Part model, mm, in its own coordinate system. A direction names the side the tool comes from. Coordinates: 2 decimals unless noted, no trailing zeros. Order: outer loops, then holes, each group sorted by start corner. A loop starts at its lowest first (then second) coordinate and runs counter-clockwise, first axis right, second up.
from build123d import *

# Parameters (mm, degrees)
F0_R           = 4.75
F1_DEPTH       = 2.5
F2_D           = 4.25
F3_D           = 4.5
F3_CSINK_D     = 7
F3_CSINK_ANGLE = 90
F4_D           = 4
F4_CBORE_D     = 7
F4_CBORE_DEPTH = 1


with BuildPart() as f1:
    # F0 (on Front) → F1 (new body)
    with BuildSketch(Plane.XZ):
        with BuildLine():
            ThreePointArc((60.5, 28.5), (59.62132, 30.62132), (57.5, 31.5))
            Line((57.5, 31.5), (-57.5, 31.5))
            ThreePointArc((-57.5, 31.5), (-59.62132, 30.62132), (-60.5, 28.5))
            Line((-60.5, 28.5), (-60.5, -28.5))
            ThreePointArc((-60.5, -28.5), (-59.62132, -30.62132), (-57.5, -31.5))
            Line((-57.5, -31.5), (57.5, -31.5))
            ThreePointArc((57.5, -31.5), (59.62132, -30.62132), (60.5, -28.5))
            Line((60.5, -28.5), (60.5, 28.5))
        make_face()
        with Locations((-44.260606, 0)):
            Circle(F0_R, mode=Mode.SUBTRACT)
        with BuildLine():
            ThreePointArc((11.989579, 27.5), (25.096687, 16.436433), (30, 0))
            ThreePointArc((30, 0), (25.096687, -16.436433), (11.989579, -27.5))
            ThreePointArc((11.989579, -27.5), (0, -30), (-11.989579, -27.5))
            ThreePointArc((-11.989579, -27.5), (-30, 0), (-11.989579, 27.5))
            ThreePointArc((-11.989579, 27.5), (0, 30), (11.989579, 27.5))
        make_face(mode=Mode.SUBTRACT)
        with BuildLine():
            Line((-11.989579, 27.5), (11.989579, 27.5))
            ThreePointArc((11.989579, 27.5), (0, 30), (-11.989579, 27.5))
        make_face()
        with BuildLine():
            ThreePointArc((-11.989579, -27.5), (0, -30), (11.989579, -27.5))
            Line((11.989579, -27.5), (-11.989579, -27.5))
        make_face()
    extrude(amount=F1_DEPTH)

    # F2 (through all)
    with Locations(Plane(origin=(0, 0, 0), x_dir=(1, 0, 0), z_dir=(0, 1, 0))):
        with Locations((-56.5, 25.75), (56.5, 25.75), (56.5, -25.75), (-56.5, -25.75)):
            Hole(F2_D / 2)

    # F3 (through all)
    with Locations(Plane(origin=(0, 0, 0), x_dir=(1, 0, 0), z_dir=(0, 1, 0))):
        with Locations((-25, 25), (25, 25), (25, -25), (-25, -25)):
            CounterSinkHole(F3_D / 2, F3_CSINK_D / 2, counter_sink_angle=F3_CSINK_ANGLE)

    # F4 (through all)
    with Locations(Plane(origin=(0, 0, 0), x_dir=(1, 0, 0), z_dir=(0, 1, 0))):
        with Locations((-44.260606, 10), (-44.260606, -10)):
            CounterBoreHole(F4_D / 2, F4_CBORE_D / 2, F4_CBORE_DEPTH)


solid = f1.part
Q1. Cut at A-A on x = -10.5. Write the cut outline in (y, z).
Results list:
outline: (-2.5, -31.5) - (0, -31.5) - (0, -27.5) - (-2.5, -27.5) - close; (-2.5, 27.5) - (0, 27.5) - (0, 31.5) - (-2.5, 31.5) - close
Q2. Pin check, flat tip, straight feed: pin 1 Ø5 at (x, z) = (-44.26, -10) entering from +Y. Stop position of the tip, or through.
Results list:
pin 1: stops at y = -1
Q3. Cut at C-C on x = -25. Write the cut outline in (y, z).
Results list:
outline: (-2.5, -31.5) - (0, -31.5) - (0, -28.5) - (-1.25, -27.25) - (-2.5, -27.25) - close; (-2.5, -22.75) - (-1.25, -22.75) - (0, -21.5) - (0, -16.58) - (-2.5, -16.58) - close; (-2.5, 16.58) - (0, 16.58) - (0, 21.5) - (-1.25, 22.75) - (-2.5, 22.75) - close; (-2.5, 27.25) - (-1.25, 27.25) - (0, 28.5) - (0, 31.5) - (-2.5, 31.5) - close
Q4. Mould opens along X. For faces 3 (the face through (-1, -2.5, -28)), 4 (the face through (60.5, -1, 0)), 5 (the face through (23.962, -1.884, 26.996)), 6 (the face through (-42.263, -1.76, -10.088)) say: pulls with the +X half, pulls with the -X half, needs draft (parallel to the pull), parting line crosses it, or undercut.
Results list:
face 3: needs draft
face 4: pulls with the +X half
face 5: undercut
face 6: undercut
Q5. Wall check: line 1 along Z through (x, y) = (56.5, -1.95) (3 decimals); line 2 along Z through (x, y) = (9, -0.7); line 3 along X through (y, z) = (-1.45, 12.5). Give the ranges that are in metal, low to high.
Results list:
line 1: z = -31.5 to -27.875, -23.625 to 23.625, 27.875 to 31.5
line 2: z = -31.5 to -27.5, 27.5 to 31.5
line 3: x = -60.5 to -27.27, 27.27 to 60.5
Q6. Which spindle directions (+Z, -Z, +X, -X, +Y, -Y) get a long thin tool onto all of the face, cutting with end or side? Do faces 1 (the face through (-43, -1, 12)), 2 (the face through (58.623, -1.268, -25.843)). Say none if no direction does.
Results list:
face 1: +Y
face 2: +Y, -Y
Q7. Cut at D-D on z = 18.5. Write the cut outline in (x, y), and give its area (3 significant figures).
Results list:
outline: (-60.5, -2.5) - (-23.62, -2.5) - (-23.62, 0) - (-60.5, 0) - close; (23.62, -2.5) - (60.5, -2.5) - (60.5, 0) - (23.62, 0) - close
area: 184 mm2
Q8. Cut at B-B on z = 10. Write the cut outline in (x, y), and give its area (3 significant figures).
Results list:
outline: (-60.5, -2.5) - (-46.26, -2.5) - (-46.26, -1) - (-47.76, -1) - (-47.76, 0) - (-60.5, 0) - close; (-42.26, -2.5) - (-28.28, -2.5) - (-28.28, 0) - (-40.76, 0) - (-40.76, -1) - (-42.26, -1) - close; (28.28, -2.5) - (60.5, -2.5) - (60.5, 0) - (28.28, 0) - close
area: 148 mm2
